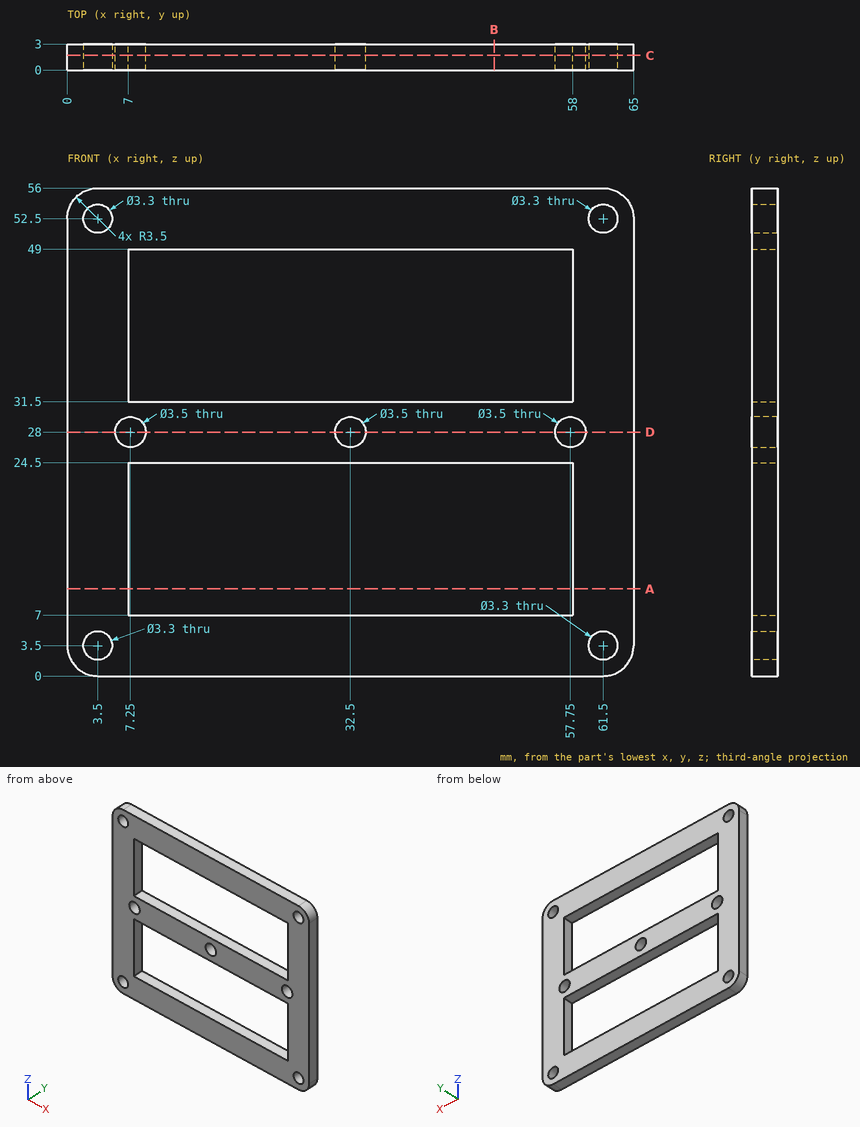
Study the drawing (mm; zero at the part's minimum x, y, z) and answer. Give positions to 0.01 mm unless a question says otherwise; leave off trailing zeros. Loops run counter-clockwise (first coordinate to the right, second up) from the corner with the lowest first, then second, coordinate; pieces in that order, holes last. Notation, with made-up numbers: (-29, 44) - (-24, 44) arc R22 ccw to (-24, 75) - close; hole circle Ø6 at (-29.5, 72). An arc over 180 degrees is marked (long way). Use CSV: the item, a comma, the result in double quotes. Start each with the question number.
(1) Find section D-D, the plane z = 28. Determine the outline of the cut face in (x, y).
(2) Find section A-A, the plane z = 10. Determine the outline of the cut face in (x, y).
(3) Find section B-B, the plane x = 49. Determine the outline of the cut face in (y, z), plus the area to 3 significant figures.
(4) Find section C-C, the plane y = 1.7. Count the separate pieces of the cut face and the enclosed holes in it, plus the area to 3 significant figures.
(5) Each of these flat-tipped pins is pushed along its axis until it touches: pin 1 (3 mm diameter, centred on x = 57.75, z = 28, fed in from -Y); pin 2 (5.5 mm diameter, centred on x = 3.5, z = 52.5, fed in from +Y). Where does it stop, or does it pass through?
(6) Find the intervals of material crossed by L1, parallel to Z at x = 48.5, y = 1.75; L2, parallel to X at y = 1.45, z = 28; L3, parallel to X at y = 2.45, z = 3.5, in increasing order.
Results found:
1,outline,"(0, 0) - (5.5, 0) - (5.5, 3) - (0, 3) - close; (9, 0) - (30.75, 0) - (30.75, 3) - (9, 3) - close; (34.25, 0) - (56, 0) - (56, 3) - (34.25, 3) - close; (59.5, 0) - (65, 0) - (65, 3) - (59.5, 3) - close"
2,outline,"(0, 0) - (7, 0) - (7, 3) - (0, 3) - close; (58, 0) - (65, 0) - (65, 3) - (58, 3) - close"
3,outline,"(0, 0) - (3, 0) - (3, 7) - (0, 7) - close; (0, 24.5) - (3, 24.5) - (3, 31.5) - (0, 31.5) - close; (0, 49) - (3, 49) - (3, 56) - (0, 56) - close"
3,area,"63.0 mm^2"
4,separate pieces,"1"
4,enclosed holes,"9"
4,area,"1,780 mm^2"
5,pin 1,"through"
5,pin 2,"y = 3"
6,L1,"0 to 7, 24.5 to 31.5, 49 to 56"
6,L2,"0 to 5.5, 9 to 30.75, 34.25 to 56, 59.5 to 65"
6,L3,"0 to 1.85, 5.15 to 59.85, 63.15 to 65"
